Design review of the part built by this model. Coordinates are the model's own, in mm. A direction names the side the tool comes from. Give positions to 0.01 mm unless a question says otherwise; leave off trailing zeros. Order: outer loops, then holes, each group sorted by start corner. A loop starts at its lowest first (then second) coordinate and runs counter-clockwise, first axis right, second up. Notation, with made-up numbers: (32.5, 2) -> (37.5, 2) arc R19 cw to (37.5, 8) -> close; hole circle Ø10 at (-19.75, 73.5). An arc over 180 degrees is marked (long way). One line per item, written item: value.
from build123d import *

# Parameters (mm, degrees)
SKETCH1_R           = 12.065
BOSS_EXTRUDE1_DEPTH = 19.812
SKETCH2_R           = 2.921
BOSS_EXTRUDE2_DEPTH = 25.4
SKETCH3_R           = 4.0005
BOSS_EXTRUDE3_DEPTH = 3.81
FILLET3_R           = 2.54
SKETCH7_R           = 2.8702
CUT_EXTRUDE1_DEPTH  = 12.7
CIRPATTERN1_COUNT   = 2
CIRPATTERN1_ANGLE   = 90
FILLET4_R           = 2.54
CUT_EXTRUDE2_REACH  = 53.907
SKETCH9_R           = 0.635


with BuildPart() as part:
    # Sketch1 → Boss-Extrude1 (new body)
    with BuildSketch(Plane(origin=(0, 0, 0), x_dir=(1, 0, 0), z_dir=(0, 1, 0))):
        with Locations(Location((0, 0, 0), (0, 0, 270))):
            Circle(SKETCH1_R)
    extrude(amount=BOSS_EXTRUDE1_DEPTH)

    # Sketch2 → Boss-Extrude2 (add)
    with BuildSketch(Plane(origin=(0, 19.812, 0), x_dir=(1, 0, 0), z_dir=(0, 1, 0))):
        with Locations(Location((0, 0, 0), (0, 0, 270))):
            Circle(SKETCH2_R)
    extrude(amount=BOSS_EXTRUDE2_DEPTH)

    # Sketch3 → Boss-Extrude3 (add)
    with BuildSketch(Plane(origin=(0, 45.212, 0), x_dir=(1, 0, 0), z_dir=(0, 1, 0))):
        with Locations(Location((0, 0, 0), (0, 0, 90))):
            Circle(SKETCH3_R)
    extrude(amount=BOSS_EXTRUDE3_DEPTH)

    # Fillet3
    fillet3_edges = [part.edges().sort_by_distance(p)[0] for p in [
        (0, 49.022, 4.0005),
    ]]
    fillet(fillet3_edges, radius=FILLET3_R)

    # Sketch7 → Cut-Extrude1 (cut, symmetric)
    with BuildSketch(Plane.XY):
        with Locations(Location((0, 7.62, 0), (0, 0, 90.000000025))):
            Circle(SKETCH7_R)
    cut_extrude1 = extrude(amount=CUT_EXTRUDE1_DEPTH, both=True, mode=Mode.SUBTRACT)

    # CirPattern1: Cut-Extrude1 ×2 about axis
    cirpattern1_axis = Axis((0, 45.212, 0), (0, -1, 0))
    for i in range(1, CIRPATTERN1_COUNT):
        add(cut_extrude1.rotate(cirpattern1_axis, i * CIRPATTERN1_ANGLE / (CIRPATTERN1_COUNT - 1)), mode=Mode.SUBTRACT)

    # Loft1: read off the stored shape, not the designer's step
    # Loft1: loft between two sections, ruled curve by curve
    loft1_from = [
        Edge.make_bspline([(4.000436037, 45.212, 0.022622174), (3.955191689, 45.212, 8.023494248), (-4.045680385, 45.212, 7.9782499), (-4.000436037, 45.212, -0.022622174), (-3.955191689, 45.212, -8.023494248), (4.045680385, 45.212, -7.9782499), (4.000436037, 45.212, 0.022622174)], [0, 0, 0, 0, 0.5, 0.5, 0.5, 1, 1, 1, 1], 3, [1, 0.333333333, 0.333333333, 1, 0.333333333, 0.333333333, 1]),
    ]
    loft1_to = [
        Edge.make_bspline([(2.781979214, 42.672, 0.890411509), (1.001156196, 42.672, 6.454369936), (-4.562802231, 42.672, 4.673546919), (-2.781979214, 42.672, -0.890411509), (-1.001156196, 42.672, -6.454369936), (4.562802231, 42.672, -4.673546919), (2.781979214, 42.672, 0.890411509)], [0, 0, 0, 0, 0.5, 0.5, 0.5, 1, 1, 1, 1], 3, [1, 0.333333333, 0.333333333, 1, 0.333333333, 0.333333333, 1]),
    ]
    loft1 = Solid(Shell([*[Face.make_surface_from_curves(loft1_from[k], loft1_to[k]) for k in range(1)], Face(Wire(loft1_from)), Face(Wire(loft1_to))]))
    add(loft1)

    # Fillet4
    fillet4_edges = [part.edges().sort_by_distance(p)[0] for p in [
        (-2.836767549, 45.212, 2.820771193),
    ]]
    fillet(fillet4_edges, radius=FILLET4_R)

    # Cut-Extrude2: up to this face of the body (flat: up to its plane)
    cut_extrude2_end = Plane(part.part.faces().sort_by_distance((0, 0, 0))[0])
    # Sketch9 → Cut-Extrude2 (cut, up to the picked face)
    with BuildSketch(Plane(origin=(0, 49.022, 0), x_dir=(1, 0, 0), z_dir=(0, 1, 0)), mode=Mode.PRIVATE) as cut_extrude2_sk1:
        with Locations(Location((0, 0, 0), (0, 0, 270))):
            Circle(SKETCH9_R)
    cut_extrude2_tool1 = split(extrude(cut_extrude2_sk1.sketch, amount=-CUT_EXTRUDE2_REACH, mode=Mode.PRIVATE), bisect_by=cut_extrude2_end, keep=Keep.BOTH, mode=Mode.PRIVATE)
    add(cut_extrude2_tool1.solids().sort_by(Axis((0, 49.022, 0), (0, -1, 0)))[0], mode=Mode.SUBTRACT)


solid = part.part
Item 1: Add section C-C on z = -6.5. Give the boundary of the cut face in (x, y), plus the area to 3 significant figures.
Returned:
outline: (-10.16, 0) -> (10.16, 0) -> (10.16, 19.81) -> (-10.16, 19.81) -> close; hole circle Ø5.74 at (0, 7.62)
area: 377 mm²
Item 2: Draft analysis for pull direction X (two halves, no side actions). For faces 3 (the cylindrical face through (-1.202, 46.126, -3.816)), 4 (the flat face through (1, 49.022, 0)), 5 (the cylindrical face through (-1.94, 5.505, -7.47)), state which applies: pulls with the +X half, pulls with the -X half, needs draft (parallel to the pull), parting line crosses it, or undercut.
Returned:
face 3: parting line crosses it
face 4: needs draft
face 5: undercut
Item 3: Clearance check with flat-ended pins moving along their axes: P1, Ø2, axis at y = 10, z = -8.5, coming from the +X side; P2, Ø2, axis at y = 28.5, z = 2, coming from the -X side; P3, Ø2, axis at x = 7, y = 14, coming from the +Z side. State where each tip first meets the part, or that it passes through.
Returned:
P1: x = 9.45
P2: x = -2.74
P3: z = 10.47
Item 4: Add section D-D on y = 41. Give the boundary of the cut face in (x, z) (3 decimals).
Returned:
outline: circle Ø5.842 at (0, 0); hole circle Ø1.27 at (0, 0)
Item 5: To check wall thickness, follow line 1 along Y through (x, z) = (0, 5.25); line 2 along X through (y, z) = (21.5, 0) (3 decimals); line 3 along X through (y, z) = (14.5, 0) (3 decimals). State the ranges of each line that lie inside material, in increasing order. Write a range as from..to.
Returned:
line 1: 0..4.75, 10.49..19.81
line 2: -2.921..-0.635, 0.635..2.921
line 3: -12.065..-0.635, 0.635..12.065
Item 6: Add section A-A on y = 7.62. Give the boundary of the cut face in (x, z) (3 decimals), plus the area to 3 significant figures.
Returned:
outline: (-11.719, -2.87) arc R12.065 ccw to (-2.87, -11.719) -> (-2.87, -2.87) -> close; (-11.719, 2.87) -> (-2.87, 2.87) -> (-2.87, 11.719) arc R12.065 ccw to start; (2.87, -11.719) arc R12.065 ccw to (11.719, -2.87) -> (2.87, -2.87) -> close; (2.87, 2.87) -> (11.719, 2.87) arc R12.065 ccw to (2.87, 11.719) -> close
area: 216 mm²
Item 7: Add section B-B on x = -7.5. Give the boundary of the cut face in (y, z), plus the area to 3 significant figures.
Returned:
outline: (0, -9.45) -> (19.81, -9.45) -> (19.81, 9.45) -> (0, 9.45) -> close; hole circle Ø5.74 at (7.62, 0)
area: 349 mm²
Item 8: Machinability: for faces 1 (the cylindrical face through (-2.42, 9.16, 6.34)), 2 (the cylindrical face through (-1.119, 31.082, 2.698)), which of the approach directions +Z, -Z, +X, -X, +Y, -Y give a long, thin tool a straight path to every point of the face, cutting with its end or side? Answer none if there is none.
Returned:
face 1: +Z, -Z
face 2: none
